Here's how the part is built. I have some questions about the finished solid (model axes, mm). Face numbers are marked on the shaded views. A direction names the side the tool comes from. Give positions to 0.01 mm unless a question says otherwise; leave off trailing zeros. Order: outer loops, then holes, each group sorted by start corner. A loop starts at its lowest first (then second) coordinate and runs counter-clockwise, first axis right, second up. Notation, with made-up numbers: (59, 25.25) - (76, 25.25) arc R15 cw to (76, 47.25) - close; hole circle Ø9 at (78, -15.75). An arc over 180 degrees is marked (long way). One line per question, with ' | ' between items.
from build123d import *

# Parameters (mm, degrees)
F1_DEPTH      = 25.4
F2_R          = 22.395901736
F3_DEPTH      = 25.4
F5_DEPTH      = 22.86
F6_R          = 6.35
F7_DEPTH      = 22.861
F9_DEPTH      = 25.4
F10_T1_DEPTH  = 25.4
F10_T3_DEPTH  = 50.8
F11_R         = 21.59
F12_DEPTH     = 25.4
F13_T4_DEPTH  = 68.3456632912
F13_S5_R      = 21.59
F13_T6_DEPTH  = 36
F13_T11_DEPTH = 68.3456632912
F13_S12_R     = 21.59
F13_T13_DEPTH = 36
F13_T18_DEPTH = 68.3456632912
F13_S19_R     = 21.59
F13_T20_DEPTH = 36
F14_R         = 12.7
F15_DEPTH     = 81.0466632912


# Not quite as in the source:
# - a fillet or chamfer that OpenCascade refuses, or shapes differently, is made with other operations: its cross-section is extruded or revolved along the edge and cut away or added


with BuildPart() as f1:
    # F0 (on Front) → F1 (new body)
    with BuildSketch(Plane.XZ):
        with BuildLine():
            Line((-62.5702434896, 0), (104.5470208636, 0))
            Line((104.5470208636, 0), (104.5470208636, 14.478))
            ThreePointArc((104.5470208636, 14.478), (102.2407796587, 20.0457587951), (96.6730208636, 22.352))
            Line((96.6730208636, 22.352), (58.5730208636, 22.352))
            Line((58.5730208636, 22.352), (58.5730208636, 73.152))
            Line((58.5730208636, 73.152), (39.5230208636, 73.152))
            ThreePointArc((39.5230208636, 73.152), (37.7930667188, 45.1601637849), (21.4736518763, 22.352))
            Line((21.4736518763, 22.352), (-62.5702434896, 22.352))
            Line((-62.5702434896, 22.352), (-62.5702434896, 0))
        make_face()
    extrude(amount=F1_DEPTH)

    # F2 (on Front) → F3 (join)
    with BuildSketch(Plane.XZ):
        with Locations((-62.223136425, 22.609276697)):
            Circle(F2_R)
    extrude(amount=F3_DEPTH)

    # F4 (on Top) → F5 (join)
    with BuildSketch(Plane.XY):
        with BuildLine():
            Line((-40.0024205446, 55.6456632912), (-40.0024205446, 0))
            Line((-40.0024205446, 0), (104.1451707114, 0))
            Line((104.1451707114, 0), (103.7883380443, 48.0822120633))
            ThreePointArc((103.7883380443, 48.0822120633), (101.536671306, 53.4337730184), (96.1685478742, 55.6456632912))
            Line((96.1685478742, 55.6456632912), (-40.0024205446, 55.6456632912))
        make_face()
    extrude(amount=F5_DEPTH)

    # F6 (on face) → F7 (cut, through all)
    with BuildSketch(Plane.XY.offset(22.86)):
        with Locations((58.6848433214, 33.2936632912)):
            Circle(F6_R)
    extrude(amount=-F7_DEPTH, mode=Mode.SUBTRACT)

    # F8 (on face) → F9 (cut)
    with BuildSketch(Plane.XZ.offset(25.4)):
        with BuildLine():
            Line((22.2823120117, 0), (22.2823120117, 23.0063465614))
            ThreePointArc((22.2823120117, 23.0063465614), (21.8796568843, 22.6771033417), (21.4736518763, 22.352))
            Line((21.4736518763, 22.352), (-4.4883051887, 22.352))
            Line((-4.4883051887, 22.352), (0, 0))
            Line((0, 0), (22.2823120117, 0))
        make_face()
    extrude(amount=-F9_DEPTH, mode=Mode.SUBTRACT)

    # F10: fillet of radius 5.08 on 3 edges, made by hand

    # F10_s2 → F10_t1 (join)
    with BuildSketch(Plane.XZ):
        with BuildLine():
            ThreePointArc((63.6530208636, 22.352), (60.0609184152, 23.8398975516), (58.5730208636, 27.432))
            Line((58.5730208636, 27.432), (58.5730208636, 22.352))
            Line((58.5730208636, 22.352), (63.6530208636, 22.352))
        make_face()
        with BuildLine():
            ThreePointArc((-40.1749339209, 26.5403301063), (-38.4354512238, 23.537383006), (-35.1738015691, 22.352))
            Line((-35.1738015691, 22.352), (-39.8287124925, 22.352))
            ThreePointArc((-39.8287124925, 22.352), (-39.9033629402, 24.4543041094), (-40.1749339209, 26.5403301063))
        make_face()
    extrude(amount=F10_T1_DEPTH)

    # F10_s4 → F10_t3 (cut)
    with BuildSketch(Plane.XZ.offset(-12.7)):
        with BuildLine():
            ThreePointArc((58.5730208636, 68.072), (57.085123312, 71.6641024484), (53.4930208636, 73.152))
            Line((53.4930208636, 73.152), (58.5730208636, 73.152))
            Line((58.5730208636, 73.152), (58.5730208636, 68.072))
        make_face()
    extrude(amount=F10_T3_DEPTH, mode=Mode.SUBTRACT)

    # F11 (on face) → F12 (join)
    with BuildSketch(Plane(origin=(0, 55.6456632912, 0), x_dir=(-1, 0, 0), z_dir=(0, 1, 0))):
        with Locations((61.4217809885, 18.6838455159)):
            Circle(F11_R)
    extrude(amount=-F12_DEPTH)

    # F13: fillet of radius 5.08 on 1 edges, made by hand


with BuildPart() as f13_tool2:
    # F13_s3 → F13_t4 (new body)
    with BuildSketch(Plane.XZ.offset(-68.3456632912)):
        with BuildLine():
            ThreePointArc((-40.0024205446, 17.78), (-38.5145229931, 21.3721024484), (-34.9224205446, 22.86))
            Line((-34.9224205446, 22.86), (-40.0024205446, 22.86))
            Line((-40.0024205446, 22.86), (-40.0024205446, 17.78))
        make_face()
    extrude(amount=F13_T4_DEPTH)

    # F13_s5 → F13_t6 (cut, symmetric)
    with BuildSketch(Plane.XZ.offset(-34.2)):
        with Locations((-61.4217809885, 18.6838455159)):
            Circle(F13_S5_R)
    extrude(amount=F13_T6_DEPTH, both=True, mode=Mode.SUBTRACT)

    split(bisect_by=Plane.XZ.offset(-30.2456632912), keep=Keep.BOTTOM)


with BuildPart() as f1_1:
    add(f1.part)

    # F13_t1: cut F13_tool2
    add(f13_tool2.part, mode=Mode.SUBTRACT)


with BuildPart() as f13_tool9:
    # F13_s10 → F13_t11 (new body)
    with BuildSketch(Plane.XZ.offset(-68.3456632912)):
        with BuildLine():
            ThreePointArc((-40.0024205446, 17.78), (-38.5145229931, 21.3721024484), (-34.9224205446, 22.86))
            Line((-34.9224205446, 22.86), (-40.0024205446, 22.86))
            Line((-40.0024205446, 22.86), (-40.0024205446, 17.78))
        make_face()
    extrude(amount=F13_T11_DEPTH)

    # F13_s12 → F13_t13 (intersect, symmetric)
    with BuildSketch(Plane.XZ.offset(-34.2)):
        with Locations((-61.4217809885, 18.6838455159)):
            Circle(F13_S12_R)
    extrude(amount=F13_T13_DEPTH, both=True, mode=Mode.INTERSECT)

    split(bisect_by=Plane.XZ.offset(-30.2456632912), keep=Keep.TOP)


with BuildPart() as f1_2:
    add(f1_1.part)

    # F13_t8: cut F13_tool9
    add(f13_tool9.part, mode=Mode.SUBTRACT)


with BuildPart() as f13_tool16:
    # F13_s17 → F13_t18 (new body)
    with BuildSketch(Plane.XZ.offset(-68.3456632912)):
        with BuildLine():
            ThreePointArc((-40.0024205446, 17.78), (-38.5145229931, 21.3721024484), (-34.9224205446, 22.86))
            Line((-34.9224205446, 22.86), (-40.0024205446, 22.86))
            Line((-40.0024205446, 22.86), (-40.0024205446, 17.78))
        make_face()
    extrude(amount=F13_T18_DEPTH)

    # F13_s19 → F13_t20 (cut, symmetric)
    with BuildSketch(Plane.XZ.offset(-34.2)):
        with Locations((-61.4217809885, 18.6838455159)):
            Circle(F13_S19_R)
    extrude(amount=F13_T20_DEPTH, both=True, mode=Mode.SUBTRACT)

    split(bisect_by=Plane.XZ.offset(-30.2456632912), keep=Keep.TOP)


with BuildPart() as f1_3:
    add(f1_2.part)

    # F13_t15: cut F13_tool16
    add(f13_tool16.part, mode=Mode.SUBTRACT)

    # F14 (on face) → F15 (cut, through all)
    with BuildSketch(Plane.XZ.offset(25.4)):
        with Locations((-62.223136425, 22.609276697)):
            Circle(F14_R)
    extrude(amount=-F15_DEPTH, mode=Mode.SUBTRACT)


solid = f1_3.part
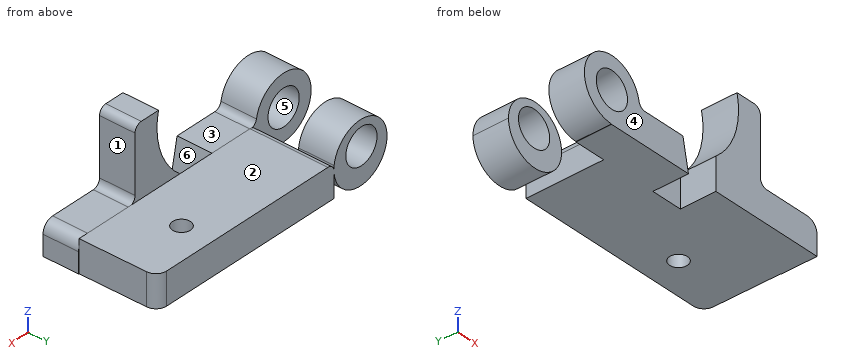
1) Please list where these lines run through material, in increasing order: L1, parallel to X at y = 34, z = 21; L2, parallel to Z at x = 8.5, y = 38; L3, parallel to X at y = 2, z = 10.
Model answer:
L1: x = -82.89 to -74.82, -49.63 to -39.96, -38.85 to 52.37, 65 to 103.89 | L2: z = 0 to 22.86 | L3: x = -40 to 104.13
2) On a 3-axis mill with a long thin cutter (end or side, diameter ignored), from which of +Z, -Z, +X, -X, +Y, -Y can I reach the whole of each face in a straight line? I mean the marked faces 1, 2 and 3. Say none if no direction works.
Model answer:
face 1: +Z, +X, +Y, -Y | face 2: +Z, +X, +Y | face 3: +Z, -Y
3) I'm going to push flat-ended pins straight in: P1, Ø11.5, axis at y = -14, z = 15.5, coming from the -X side; P2, Ø10, axis at x = -60, y = 27, coming from the +Z side; P3, Ø11.5, axis at x = 58.68, y = 33.29, coming from the +Z side; P4, Ø10, axis at x = -9.5, y = 30, coming from the -Z side. Where does each tip first touch, or does it pass through?
Model answer:
P1: stops at x = -84.58 | P2: stops at z = 40.27 | P3: passes through | P4: stops at z = 0
4) I want a section at B-B (x = -54). List the corners of the cut face in (y, z) for me, plus the area to 3 significant figures.
Model answer:
outline: (-25.4, 0) - (0, 0) - (0, 12.93) - (-25.4, 12.93) - close; (-25.4, 32.29) - (0, 32.29) - (0, 43.44) - (-25.4, 43.44) - close; (30.25, -1.59) - (55.65, -1.59) - (55.65, 12.93) - (30.25, 12.93) - close; (30.25, 32.29) - (55.65, 32.29) - (55.65, 38.96) - (30.25, 38.96) - close | area: 1,150 mm2
5) I want a section at A-A (y = -2). List the corners of the cut face in (x, z) for me, plus the area to 3 significant figures.
Model answer:
outline: (-62.57, 0) - (0, 0) - (-4.49, 22.35) - (-35.17, 22.35) arc R5.08 cw to (-40.17, 26.54) arc R22.4 ccw (long way) to (-62.57, 0.22) - close; (22.28, 0) - (104.55, 0) - (104.55, 14.48) arc R7.87 ccw to (96.67, 22.35) - (63.65, 22.35) arc R5.08 cw to (58.57, 27.43) - (58.57, 68.07) arc R5.08 ccw to (53.49, 73.15) - (39.52, 73.15) arc R50.8 cw to (22.28, 23.01) - close; hole circle Ø25.4 at (-62.22, 22.61) | area: 4,990 mm2
6) Thinking about a two-plate mould opening in Z: for the marked faces 4, 5 and 6, which applies, +Z half, -Z half, draft (parallel to the pull), parting line (faces both ways), or undercut?
Model answer:
face 4: draft | face 5: undercut | face 6: +Z half
7) I want a section at C-C (x = 4.5). List the corners of the cut face in (y, z) for me.
Model answer:
outline: (0, 0) - (55.65, 0) - (55.65, 22.86) - (0, 22.86) - close
8) I want a section at D-D (y = 50). List the corners of the cut face in (x, z) for me.
Model answer:
outline: (-40, 0) - (103.53, 0) - (103.53, 22.86) - (-34.92, 22.86) arc R5.08 ccw to (-39.84, 19.07) arc R21.59 ccw (long way) to (-40, 15.97) - close; hole circle Ø25.4 at (-62.22, 22.61)
